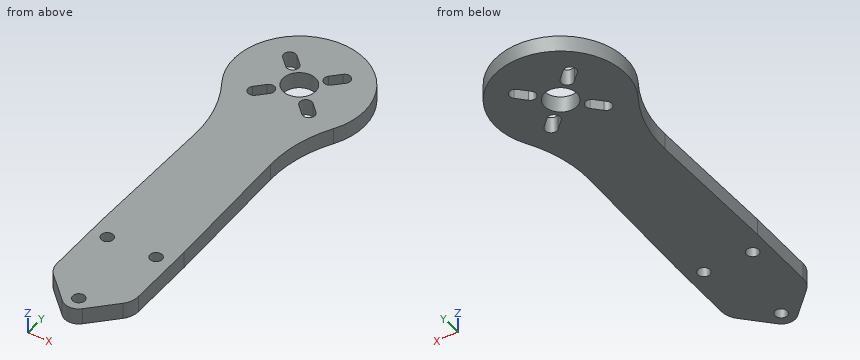
from build123d import *

# Parameters (mm, degrees)
F0_R     = 1.5
F0_R_2   = 4
F1_DEPTH = 4
F2_R     = 5
F3_R     = 32


# Not quite as in the source:
# - a feature names something its author has since deleted; it is built from what else it names


with BuildPart() as f1:
    # F0 (on Top) → F1 (new body)
    with BuildSketch(Plane.XY):
        with BuildLine():
            Line((-9, 91.7712434447), (-10, 46))
            Line((-10, 46), (-10, 26.6170093579))
            Line((-10, 26.6170093579), (-2.4748737342, 19.091883092))
            ThreePointArc((-2.4748737342, 19.091883092), (0, 18.0667568262), (2.4748737342, 19.091883092))
            Line((2.4748737342, 19.091883092), (10, 26.6170093579))
            Line((10, 26.6170093579), (10, 46))
            Line((10, 46), (9, 91.7712434447))
            ThreePointArc((9, 91.7712434447), (0, 121), (-9, 91.7712434447))
        make_face()
        with Locations((-6, 41.5667568262)):
            Circle(F0_R, mode=Mode.SUBTRACT)
        with Locations((0, 21.5667568262)):
            Circle(F0_R, mode=Mode.SUBTRACT)
        with Locations((6, 41.5667568262)):
            Circle(F0_R, mode=Mode.SUBTRACT)
        with BuildLine():
            ThreePointArc((-5.6568542495, 101.4644660941), (-3.5355339059, 101.4644660941), (-3.5355339059, 99.3431457505))
            Line((-3.5355339059, 99.3431457505), (-5.6568542495, 97.2218254069))
            ThreePointArc((-5.6568542495, 97.2218254069), (-7.7781745931, 97.2218254069), (-7.7781745931, 99.3431457505))
            Line((-7.7781745931, 99.3431457505), (-5.6568542495, 101.4644660941))
        make_face(mode=Mode.SUBTRACT)
        with BuildLine():
            ThreePointArc((-3.5355339059, 110.6568542495), (-3.5355339059, 108.5355339059), (-5.6568542495, 108.5355339059))
            Line((-5.6568542495, 108.5355339059), (-7.7781745931, 110.6568542495))
            ThreePointArc((-7.7781745931, 110.6568542495), (-7.7781745931, 112.7781745931), (-5.6568542495, 112.7781745931))
            Line((-5.6568542495, 112.7781745931), (-3.5355339059, 110.6568542495))
        make_face(mode=Mode.SUBTRACT)
        with Locations((0, 105)):
            Circle(F0_R_2, mode=Mode.SUBTRACT)
        with BuildLine():
            ThreePointArc((3.5355339059, 99.3431457505), (3.5355339059, 101.4644660941), (5.6568542495, 101.4644660941))
            Line((5.6568542495, 101.4644660941), (7.7781745931, 99.3431457505))
            ThreePointArc((7.7781745931, 99.3431457505), (7.7781745931, 97.2218254069), (5.6568542495, 97.2218254069))
            Line((5.6568542495, 97.2218254069), (3.5355339059, 99.3431457505))
        make_face(mode=Mode.SUBTRACT)
        with BuildLine():
            ThreePointArc((5.6568542495, 108.5355339059), (3.5355339059, 108.5355339059), (3.5355339059, 110.6568542495))
            Line((3.5355339059, 110.6568542495), (5.6568542495, 112.7781745931))
            ThreePointArc((5.6568542495, 112.7781745931), (7.7781745931, 112.7781745931), (7.7781745931, 110.6568542495))
            Line((7.7781745931, 110.6568542495), (5.6568542495, 108.5355339059))
        make_face(mode=Mode.SUBTRACT)
    extrude(amount=F1_DEPTH)

    # F2
    f2_edges = [f1.edges().sort_by_distance(p)[0] for p in [
        (10, 46, 2),
        (-10, 46, 2),
        (-10, 26.617009, 2),
        (10, 26.617009, 2),
    ]]
    fillet(f2_edges, radius=F2_R)

    # F3
    f3_edges = [f1.edges().sort_by_distance(p)[0] for p in [
        (-9, 91.771243, 2),
        (9, 91.771243, 2),
    ]]
    fillet(f3_edges, radius=F3_R)


solid = f1.part
CAD build for the part. Positions are in the model's coordinates, mm. Coordinates: 2 decimals unless noted, no trailing zeros. Write each loop counter-clockwise with the first axis right and the second up, starting at its lowest first coordinate (ties: lowest second). Pieces come first, ordered by that corner, then holes. Notation, with made-up numbers: (-14.75, 35) - (1.25, 35) arc R17 ccw to (1.25, 67) - close; hole circle Ø8 at (51, -29). An arc over 180 degrees is marked (long way). Use a Markdown table: item, result. Add a question column.
Item 1: Band-saw the part on B-B, the plane z = 1.85. Give the number of separate pieces and of enclosed holes in the cut face, and give its area (3 significant figures).
Item 2: Band-saw the part on D-D, the plane x = -12. Give the cut face in (y, z), and give its area (3 significant figures).
Item 3: Flat gauge pin, fed straight in: pin 1 (1.8 mm diameter, centred on x = -6, y = 41.57, fed in from +Z). Where does the tip first touch, or does it go through?
Item 4: Band-saw the part on A-A, the plane x = 0. Give the cut face in (y, z).
Item 5: Drill centre lines: L1, parallel to Y at x = 0, z = 1.45; L2, parallel to X at y = 41.5, z = 1.6; L3, parallel to Y at x = -6, z = 2.45. Where is each one in solid material? Low to high. Write a range as from..to.
Item 6: Band-saw the part on C-C, the plane y = 63. Give the cut face in (x, z), and give its area (3 significant figures).
Numbers:
| question | item | result |
|---|---|---|
| 1 | separate pieces | 1 |
| 1 | enclosed holes | 8 |
| 1 | area | 2,010 mm2 |
| 2 | outline | (93.43, 0) - (115.58, 0) - (115.58, 4) - (93.43, 4) - close |
| 2 | area | 88.6 mm2 |
| 3 | pin 1 | through |
| 4 | outline | (18.07, 0) - (20.07, 0) - (20.07, 4) - (18.07, 4) - close; (23.07, 0) - (101, 0) - (101, 4) - (23.07, 4) - close; (109, 0) - (121, 0) - (121, 4) - (109, 4) - close |
| 5 | L1 | 18.07..20.07, 23.07..101, 109..121 |
| 5 | L2 | -10..-7.5, -4.5..4.5, 7.5..10 |
| 5 | L3 | 22.62..40.07, 43.07..96.97, 101.12..108.88, 113.03..119.83 |
| 6 | outline | (-9.63, 0) - (9.63, 0) - (9.63, 4) - (-9.63, 4) - close |
| 6 | area | 77.0 mm2 |
